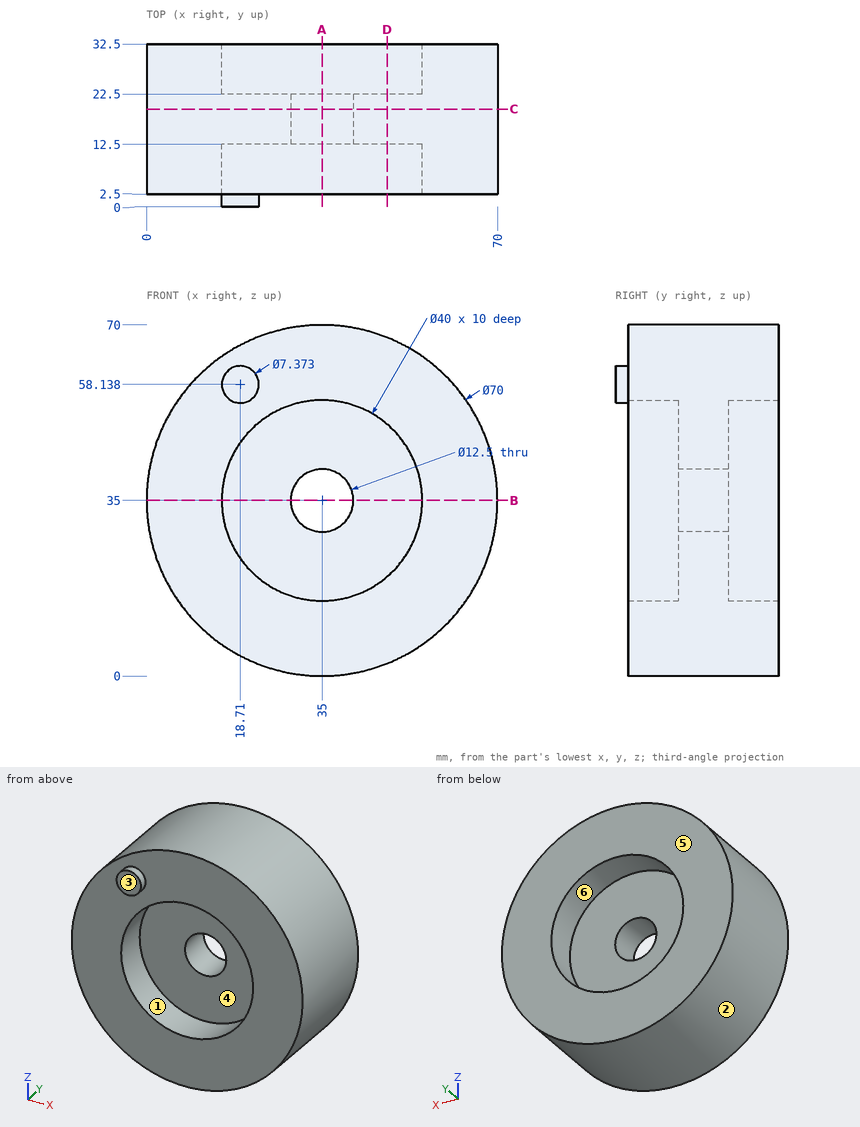
The figure shows three views and two pictorial views of one solid part (mm, origin at its lowest corner). Answer the questions. A direction names the side the tool comes from. Give positions to 0.01 mm unless a question says otherwise; leave off trailing zeros. Loops run counter-clockwise (first coordinate to the right, second up) from the corner with the lowest first, then second, coordinate; pieces in that order, holes last. Notation, with made-up numbers: M 21,-12 L 57,-12 A26 cw 57,25 Z; hole C 66,1.5 d5. An arc over 180 degrees is marked long. Write each question's results on one line, items separated by ' | '.
1. Section A-A on x = 35 is taken. Give the vertices of the cut face in (y, z).
Values:
outline: M 2.5,0 L 32.5,0 L 32.5,15 L 22.5,15 L 22.5,28.75 L 12.5,28.75 L 12.5,15 L 2.5,15 Z; M 2.5,55 L 12.5,55 L 12.5,41.25 L 22.5,41.25 L 22.5,55 L 32.5,55 L 32.5,70 L 2.5,70 Z
2. Given pin 1 (24 mm diameter, centred on x = 35, z = 35, fed in from +Y); pin 2 (1.5 mm diameter, centred on y = 8.5, z = 23.5, fed in from +X); pin 3 (1.5 mm diameter, centred on x = 41, y = 4, fed in from -Z), each flat-ended and moving along its own axis, determine where each tip first touches the part or whether it passes through.
Values:
pin 1: stops at y = 22.5 | pin 2: stops at x = 68.31 | pin 3: stops at z = 0.4
3. Section D-D on x = 48 is taken. Give the vertices of the cut face in (y, z), plus the area to 3 significant figures.
Values:
outline: M 2.5,2.5 L 32.5,2.5 L 32.5,19.8 L 22.5,19.8 L 22.5,50.2 L 32.5,50.2 L 32.5,67.5 L 2.5,67.5 L 2.5,50.2 L 12.5,50.2 L 12.5,19.8 L 2.5,19.8 Z | area: 1,340 mm^2
4. A tool of negligible diameter and unlimited length cuts with its end or side. For the marked faces 4, 5 and 6, from which of +Z, -Z, +X, -X, +Y, -Y can it reach the whole face along a straight path? Write none if from no direction.
Values:
face 4: -Y | face 5: +Z, -Z, +X, -X, +Y | face 6: +Y
5. The mould has two halves that part along X. Classify the marked faces 1, 2 and 3: pulls with the +X half, pulls with the -X half, needs draft (parallel to the pull), parting line crosses it, or undercut.
Values:
face 1: undercut | face 2: parting line crosses it | face 3: needs draft
6. Section C-C on y = 19.5 is taken. Give the vertices of the cut face in (x, z).
Values:
outline: C 35,35 d70; hole C 35,35 d12.5
7. Straight lines are drawn through the part: line 1 (Z direction, x = 35, y = 18); line 2 (Z direction, x = 35, y = 8); line 3 (Y direction, x = 43, z = 36). For each, find the intervals that lie inside material, in ascending order. Write a range as [from, to].
Values:
line 1: z = [0, 28.75], [41.25, 70] | line 2: z = [0, 15], [55, 70] | line 3: y = [12.5, 22.5]
8. Section B-B on z = 35 is taken. Give the vertices of the cut face in (x, y).
Values:
outline: M 0,2.5 L 15,2.5 L 15,12.5 L 28.75,12.5 L 28.75,22.5 L 15,22.5 L 15,32.5 L 0,32.5 Z; M 41.25,12.5 L 55,12.5 L 55,2.5 L 70,2.5 L 70,32.5 L 55,32.5 L 55,22.5 L 41.25,22.5 Z
